Could you check a few things on this model? Use its own coordinates, in mm. Face numbers are marked on the shaded views. A direction names the side the tool comes from. Give positions to 0.01 mm unless a question says otherwise; leave off trailing zeros. Write each loop counter-clockwise with the first axis right and the second up, starting at its lowest first coordinate (ties: lowest second). Pieces come first, ordered by that corner, then holes. Notation, with made-up numbers: (-3.75, -39.5) - (28.25, -39.5) arc R5 ccw to (28.25, -31.5) - close; hole circle Ø2 at (81.25, 56). An arc over 180 degrees is marked (long way). Write item = value, one per line.
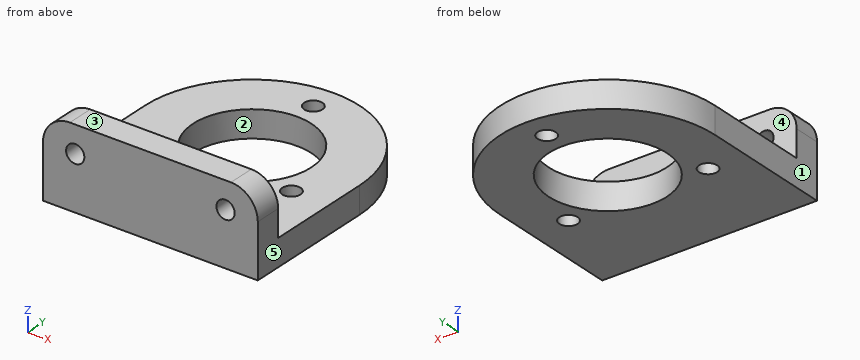
from build123d import *

# Parameters (mm, degrees)
SKETCH1_R            = 11
BOSS_EXTRUDE1_DEPTH  = 5
M3_CLEARANCE_HOLE1_D = 3.4
CIRPATTERN1_COUNT    = 3
SKETCH5_W            = 40
SKETCH5_H            = 5
BOSS_EXTRUDE2_DEPTH  = 15
M3_CLEARANCE_HOLE3_D = 3.4
FILLET1_R            = 5


with BuildPart() as part:
    # Sketch1 → Boss-Extrude1 (new body)
    with BuildSketch(Plane.XY):
        with BuildLine():
            Line((-20, -4.3e-08), (-20, -20))
            Line((-20, -20), (20, -20))
            Line((20, -20), (20, 0))
            ThreePointArc((20, 0), (-2.2e-08, 20), (-20, -4.3e-08))
        make_face()
        Circle(SKETCH1_R, mode=Mode.SUBTRACT)
    extrude(amount=BOSS_EXTRUDE1_DEPTH)

    # M3 Clearance Hole1 (through all)
    with Locations(Plane(origin=(0, 15, 5), x_dir=(1, 0, 0), z_dir=(0, 0, 1))):
        with Locations((0, 0)):
            m3_clearance_hole1 = Hole(M3_CLEARANCE_HOLE1_D / 2)

    # CirPattern1: M3 Clearance Hole1 ×3 about axis
    cirpattern1_axis = Axis((0, 0, 0), (0, 0, 1))
    for i in range(1, CIRPATTERN1_COUNT):
        add(m3_clearance_hole1.rotate(cirpattern1_axis, i * 360 / CIRPATTERN1_COUNT), mode=Mode.SUBTRACT)

    # Sketch5 → Boss-Extrude2 (add)
    with BuildSketch(Plane.XY):
        with Locations((0, -22.5)):
            Rectangle(SKETCH5_W, SKETCH5_H)
    extrude(amount=BOSS_EXTRUDE2_DEPTH)

    # M3 Clearance Hole3 (through all)
    with Locations(Plane(origin=(-14, -20, 10), x_dir=(0, 0, 1), z_dir=(0, 1, 0))):
        with Locations((0, 0), (0, 28)):
            Hole(M3_CLEARANCE_HOLE3_D / 2)

    # Fillet1
    fillet1_edges = [part.edges().sort_by_distance(p)[0] for p in [
        (-20, -22.5, 15),
        (20, -22.5, 15),
    ]]
    fillet(fillet1_edges, radius=FILLET1_R)


solid = part.part
1. If we section it at A-A, the plane x = 0: Please give me the cut outline in (y, z).
Filled sheet:
outline = (-25, 0) - (-11, 0) - (-11, 5) - (-20, 5) - (-20, 15) - (-25, 15) - close; (11, 0) - (13.3, 0) - (13.3, 5) - (11, 5) - close; (16.7, 0) - (20, 0) - (20, 5) - (16.7, 5) - close
2. If we section it at B-B, the plane y = -7.5: Please give me the cut outline in (x, z), and give its area (3 significant figures).
Filled sheet:
outline = (-20, 0) - (-14.69, 0) - (-14.69, 5) - (-20, 5) - close; (-11.29, 0) - (-8.05, 0) - (-8.05, 5) - (-11.29, 5) - close; (8.05, 0) - (11.29, 0) - (11.29, 5) - (8.05, 5) - close; (14.69, 0) - (20, 0) - (20, 5) - (14.69, 5) - close
area = 85.5 mm2
3. If we section it at D-D, the plane z = 4.25: Please give me the cut outline in (x, y).
Filled sheet:
outline = (-20, -25) - (20, -25) - (20, 0) arc R20 ccw to (-20, 0) - close; hole circle Ø3.4 at (-12.99, -7.5); hole circle Ø22 at (0, 0); hole circle Ø3.4 at (0, 15); hole circle Ø3.4 at (12.99, -7.5)
4. I need wall thicknesses on line 1 (X direction, y = -23.4, z = 10); line 2 (Y direction, x = 0.5, z = 4.25); line 3 (Y direction, x = -3, z = 11.75). Which ranges of each line are inside material? Lowest first, please.
Filled sheet:
line_1 = -20 to -15.7, -12.3 to 12.3, 15.7 to 20
line_2 = -25 to -10.99, 10.99 to 13.38, 16.62 to 19.99
line_3 = -25 to -20
5. Which directions (+Z, -Z, +X, -X, +Y, -Y) give clear straight access to the entire face, cutting with the end or side of a thin tool? Please do the marked faces 4 and 5.
Filled sheet:
face_4 = +Z, +X, -X, +Y
face_5 = +Z, -Z, +X, +Y, -Y
6. Thinking about a two-plate mould opening in X: for the marked faces 1, 2 and 3, which applies, pulls with the +X half, pulls with the -X half, needs draft (parallel to the pull), parting line crosses it, or undercut?
Filled sheet:
face_1 = pulls with the -X half
face_2 = undercut
face_3 = needs draft
7. If we section it at C-C, the plane x = -7: Please give me the cut outline in (y, z) (3 decimals).
Filled sheet:
outline = (-25, 0) - (-8.485, 0) - (-8.485, 5) - (-20, 5) - (-20, 15) - (-25, 15) - close; (8.485, 0) - (18.735, 0) - (18.735, 5) - (8.485, 5) - close
8. For pin 1 (1.5 mm diameter, centred on x = 15.5, y = 2.5, fed in from +Z); pin 2 (5 mm diameter, centred on x = -9, z = 10.5, fed in from +Y); pin 3 (6 mm diameter, centred on x = -8, z = 5, fed in from +Y), each with a flat end and sliding along its axis, tell me the tip position at first contact or that it passes through.
Filled sheet:
pin_1 = 5
pin_2 = -20
pin_3 = 19.36
